Autodesk Inventor part; units mm, degrees
ref_plane "YZ Plane" through (0, 0, 0) normal (1, 0, 0) x (0, 1, 0)
ref_plane "XZ Plane" through (0, 0, 0) normal (0, 1, 0) x (-1, 0, 0)
ref_plane "XY Plane" through (0, 0, 0) normal (0, 0, 1) x (1, 0, 0)
sketch "Sketch1" plane through (0, 0, 0) normal (0, 1, 0) x (-1, 0, 0)
  line L0 (75, 59) -> (-75, 59)
  line L1 (-75, 59) -> (-75, -59)
  line L2 (-75, -59) -> (75, -59)
  line L3 (75, -59) -> (75, 59)
  line L4 (75, 59) -> (-75, -59) construction
  line L5 (-75, 59) -> (75, -59) construction
  line L6 (62.0096, 59) -> (62.0096, -65)
  line L7 (105, 0) -> (-105, 0)
  line L8 (0, -90) -> (0, 85)
  line L9 (-62.0096, 59) -> (-62.0096, -65)
  line L10 (61.6096, 59) -> (61.6096, -59)
  line L11 (-61.6096, 59) -> (-61.6096, -59)
  line L12 (-71, 55) -> (71, 55)
  line L13 (71, 55) -> (71, -55)
  line L14 (71, -55) -> (-71, -55)
  line L15 (-71, -55) -> (-71, 55)
  line L16 (61.6096, 55) -> (53.6096, 55)
  line L17 (53.6096, 55) -> (53.6096, 47)
  line L18 (53.6096, 47) -> (61.6096, 47)
  line L19 (61.6096, 47) -> (61.6096, 55)
  line L20 (61.6096, -55) -> (53.6096, -55)
  line L21 (53.6096, -55) -> (53.6096, -47)
  line L22 (53.6096, -47) -> (61.6096, -47)
  line L23 (-61.6096, 55) -> (-53.6096, 55)
  line L24 (-53.6096, 55) -> (-53.6096, 47)
  line L25 (-53.6096, 47) -> (-61.6096, 47)
  line L26 (-61.6096, 47) -> (-61.6096, 55)
  line L27 (-53.6096, -55) -> (-53.6096, -47)
  line L28 (-53.6096, -47) -> (-61.6096, -47)
  line L29 (-61.6096, -55) -> (-53.6096, -55)
  line L30 (-61.6096, 12) -> (-53.6096, 12)
  line L31 (-53.6096, 12) -> (-53.6096, 20)
  line L32 (-53.6096, 20) -> (-61.6096, 20)
  line L33 (-61.6096, 20) -> (-61.6096, 12)
  line L34 (-61.6096, -12) -> (-53.6096, -12)
  line L35 (-53.6096, -12) -> (-53.6096, -20)
  line L36 (-53.6096, -20) -> (-61.6096, -20)
  circle A0 centre (57.6096, 51) radius 1.55
  line L37 (61.6096, 51) -> (53.6096, 51)
  line L38 (57.6096, 55) -> (57.6096, 47)
  circle A1 centre (57.6096, -51) radius 1.55
  circle A2 centre (-57.6096, 51) radius 1.55
  circle A3 centre (-57.6096, -51) radius 1.55
  line L39 (-53.6096, 16) -> (-61.6096, 16)
  line L40 (-57.6096, 20) -> (-57.6096, 12)
  circle A4 centre (-57.6096, 16) radius 1.55
  circle A5 centre (-57.6096, -16) radius 1.55
  line L41 (53.6096, 51) -> (-53.6096, 51)
  line L42 (57.6096, 47) -> (57.6096, -47)
  line L43 (53.6096, -51) -> (-53.6096, -51)
  line L44 (-57.6096, -47) -> (-57.6096, -20)
  line L45 (-57.6096, -12) -> (-57.6096, 12)
  line L46 (-57.6096, 20) -> (-57.6096, 47)
  line L47 (53.6096, 47) -> (-53.6096, -47)
  line L48 (-53.6096, 47) -> (53.6096, -47)
  line L49 (0, 0) -> (57.6096, 0)
  line L50 (0, 0) -> (-57.6096, 0)
  line L51 (0, 0) -> (-53.6096, 16)
  line L52 (0, 0) -> (-53.6096, -16)
  circle A6 centre (0, 0) radius 6
  line L53 (53.6096, 48.9948) -> (3.3795, 4.9577)
  line L54 (53.6096, 52.5) -> (-53.6096, 52.5)
  line L55 (59.1096, 47) -> (59.1096, -47)
  line L56 (53.6096, -52.5) -> (-53.6096, -52.5)
  line L57 (-59.1096, -47) -> (-59.1096, -20)
  line L58 (-59.1096, -12) -> (-59.1096, 12)
  line L59 (-59.1096, 20) -> (-59.1096, 47)
  line L60 (-55.885, 47) -> (-5.3572, 2.7019)
  line L61 (-5.9958, 0.2241) -> (-53.6096, 14.4346)
  line L62 (-53.6096, -17.5654) -> (-5.1378, -3.0988)
  line L63 (-3.3795, -4.9577) -> (-53.6096, -48.9948)
  line L64 (5.8095, -1.5) -> (57.6096, -1.5)
  line L65 (56.1096, 47) -> (56.1096, -47)
  line L66 (53.6096, 49.5) -> (-53.6096, 49.5)
  line L67 (55.5873, 46.739) -> (5.3572, 2.7019)
  line L68 (5.8095, 1.5) -> (57.6096, 1.5)
  line L69 (-53.9073, 49.2558) -> (-3.3795, 4.9577)
  line L70 (-5.1378, 3.0988) -> (-52.7517, 17.3093)
  line L71 (-5.3572, -2.7019) -> (-55.5873, -46.739)
  line L72 (53.6096, -49.5) -> (-53.6096, -49.5)
  line L73 (-56.1096, -47) -> (-56.1096, -20)
  line L74 (-56.1096, -12) -> (-56.1096, 12)
  line L75 (-56.1096, 20) -> (-56.1096, 47)
  line L76 (-54.4676, -14.6907) -> (-5.9958, -0.2241)
  line L77 (3.3795, -4.9577) -> (53.6096, -48.9948)
  line L78 (5.3572, -2.7019) -> (55.5873, -46.739)
  line L79 (1.5, 49.5) -> (1.5, 5.8095)
  line L80 (-1.5, 49.5) -> (-1.5, 5.8095)
  line L81 (1.5, -49.5) -> (1.5, -5.8095)
  line L82 (-1.5, -49.5) -> (-1.5, -5.8095)
  line L83 (-52.7517, 17.3093) -> (-53.6096, 17.5654)
  line L84 (55.5873, -46.739) -> (55.885, -47)
  line L85 (55.5873, 46.739) -> (55.885, 47)
  line L86 (-55.5873, -46.739) -> (-58.8433, -49.5936)
  point P0 (-53.6096, 55)
  point P1 (-61.6096, 55)
  point P2 (-61.6096, 47)
  point P3 (-61.6096, 0)
  point P4 (-71, 0)
  point P5 (53.6096, 55)
  point P6 (4.5116, -3.9554)
  point P7 (56.1096, -1.5)
  point P8 (-4.5116, -3.9554)
  point P9 (-56.1096, -20)
  point P10 (1.5, -49.5)
  point P11 (1.5, -5.8095)
  point P12 (-1.5, -5.8095)
  point P13 (-1.5, -49.5)
  point P14 (-1.5, 5.8095)
  point P15 (-3.3795, 4.9577)
  point P16 (-53.6096, 48.9948)
  point P17 (-1.5, 49.5)
  point P18 (56.1096, 1.5)
  point P19 (4.5116, 3.9554)
  point P20 (-53.6096, -14.4346)
  point P21 (-5.7494, 1.7159)
  point P22 (-61.6096, -47)
  point P23 (-61.6096, -55)
  point P24 (-53.6096, -55)
  point P25 (53.6096, -55)
  point P26 (61.6096, -55)
  point P27 (61.6096, -47)
  point P28 (61.6096, 47)
  point P29 (5.3572, -2.7019)
  point P30 (-55.885, -47)
  point P31 (-6.1568, -3.4029)
  point P32 (5.3572, 2.7019)
  point P33 (-6.1568, 3.4029)
  dimension "d13" = 12
  dimension "d0" = 150
  dimension "d1" = 118
  dimension "d2" = 12.9904
  dimension "d3" = 0.4
  dimension "d4" = 4
  dimension "d5" = 8
  dimension "d6" = 8
  dimension "d7" = 8
  dimension "d8" = 8
  dimension "d9" = 12
  dimension "d10" = 3.1
  dimension "d11" = 3.1
  dimension "d14" = 3
  dimension "d15" = 3
  dimension "d16" = 3
  dimension "d17" = 3
  dimension "d18" = 3
  dimension "d19" = 3
  dimension "d20" = 3
  dimension "d21" = 3
  dimension "d22" = 3
  dimension "d23" = 3
  dimension "d24" = 3
  dimension "d25" = 3
extrude "Extrusion1" add sketch "Sketch1" along normal blind 3 contours L10 L37 A0 L38 L12 | L10 L18 L38 A0 L37 | L38 A0 L37 L17 L12 | L12 L24 L25 L11 | L54 L17 L41 L8 | L8 L41 L24 L54 | L14 L21 L22 L10 | L55 L22 L42 L7 | L7 L42 L18 L55 | L41 L17 L66 L8 | L8 L66 L24 L41 | L38 L18 L17 L37 A0 | L42 L64 L65 L7 | L7 L65 L68 L42 | L32 L40 A4 L39 L11 | L25 L46 L32 L59 | L66 L79 A6 L8 | L8 A6 L80 L66 | L42 L68 L65 L18 | L56 L8 L43 L21 | L65 L64 A6 L7 | L7 A6 L68 L65 | L42 L22 L65 L64 | L11 L28 L27 L14 | L56 L27 L43 L8 | L39 A4 L40 L30 L11 | L25 L75 L32 L46 | A6 L47 L8 | L8 L48 A6 | L43 L8 L72 L21 | A6 L48 L7 | L7 L47 A6 | L43 L27 L72 L8 | L58 L30 L45 L7 | L7 L45 L34 L58 | L34 L35 L36 L11 | L32 L31 L39 A4 L40 | L52 A6 L7 | L48 A6 L8 | L8 A6 L47 | L51 A6 L48 | L7 A6 L51 | L47 A6 L52 | L17 L47 A6 L53 | L69 A6 L48 L24 | L85 L67 A6 L47 L18 | L22 L48 A6 L78 L84 | L57 L36 L44 L28 | L72 L82 A6 L8 | L8 A6 L81 L72 | L45 L30 L74 L7 | L7 L74 L34 L45 | A4 L39 L31 L30 L40 | L25 L48 A6 L70 L60 | A6 L63 L27 L47 | L47 L28 L86 L71 L62 A6 | L48 L21 L77 A6 | A6 L61 L31 L51 | L51 L31 L83 L70 L60 A6 | A6 L71 L62 L35 L52 | L52 L35 L76 A6 | L44 L36 L73 L28 | L70 A6 L60 | L62 L71 A6
equation "\"d0\" = BodyLength"
equation "\"d1\" = BodyWidth"
equation "\"d2\" = 0.433013 * BodyHeight"
equation "\"d4\" = SideThickness"
equation "\"d5\" = M3ScrewInsertBrim"
equation "\"d6\" = M3ScrewInsertBrim"
equation "\"d7\" = M3ScrewInsertBrim"
equation "\"d8\" = M3ScrewInsertBrim"
equation "\"d10\" = M3ScrewDia"
equation "\"d11\" = M3ScrewDia"
equation "\"SideThickness_1\" = 4"
equation "\"M3ScrewInsertBrim_1\" = 8"
equation "\"M3ScrewDia_1\" = 3.1"
properties part number "HexScrewGuideV2"
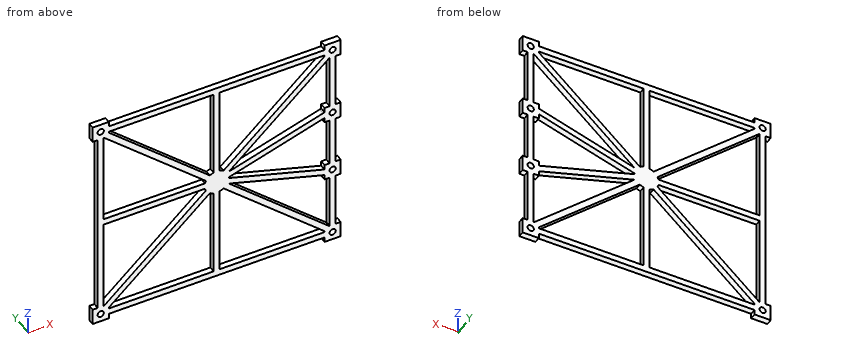
Part model, mm, in its own coordinate system. Coordinates: 2 decimals unless noted, no trailing zeros. Order: outer loops, then holes, each group sorted by start corner. A loop starts at its lowest first (then second) coordinate and runs counter-clockwise, first axis right, second up.
(1) Slice it at D-D, the plane x = 26. Write the cut outline in (y, z), and give its area (3 significant figures).
Check sheet entries:
outline: (0, -52.5) - (3, -52.5) - (3, -49.5) - (0, -49.5) - close; (0, -24.79) - (3, -24.79) - (3, -20.8) - (0, -20.8) - close; (0, -9.33) - (3, -9.33) - (3, -6.19) - (0, -6.19) - close; (0, 6.19) - (3, 6.19) - (3, 9.33) - (0, 9.33) - close; (0, 20.8) - (3, 20.8) - (3, 24.79) - (0, 24.79) - close; (0, 49.5) - (3, 49.5) - (3, 52.5) - (0, 52.5) - close
area: 60.7 mm2
(2) Slice it at C-C, the plane z = 22. Write the cut outline in (x, y), and give its area (3 significant figures).
Check sheet entries:
outline: (-59.11, 0) - (-56.11, 0) - (-56.11, 3) - (-59.11, 3) - close; (-27.37, 0) - (-22.82, 0) - (-22.82, 3) - (-27.37, 3) - close; (-1.5, 0) - (1.5, 0) - (1.5, 3) - (-1.5, 3) - close; (22.82, 0) - (27.37, 0) - (27.37, 3) - (22.82, 3) - close; (56.11, 0) - (59.11, 0) - (59.11, 3) - (56.11, 3) - close
area: 54.3 mm2
(3) Slice it at A-A, the plane z = -51. Write the cut outline in (x, y), and give its area (3 significant figures).
Check sheet entries:
outline: (-61.61, 0) - (-59.16, 0) - (-59.16, 3) - (-61.61, 3) - close; (-56.06, 0) - (56.06, 0) - (56.06, 3) - (-56.06, 3) - close; (59.16, 0) - (61.61, 0) - (61.61, 3) - (59.16, 3) - close
area: 351 mm2
(4) Pin check, flat tips, straight feed: pin 1 Ø0.9 at (y, z) = (2, 17) entering from -X; pin 2 Ø1.5 at (y, z) = (1, -37) entering from +X; pin 3 Ø1.5 at (x, y) = (16.5, 1) entering from -Z. Stop position of each tip, or through.
Check sheet entries:
pin 1: stops at x = -59.11
pin 2: stops at x = 59.11
pin 3: stops at z = -52.5
(5) Probe L1, parallel to Z at x = 46.5, y = 0.55; L2, parallel to X at y = 1.95, z = -37.5; L3, parallel to Z at x = 17.5, y = 0.5. List the from-to ranges inside material, lowest first.
Check sheet entries:
L1: z = -52.5 to -49.5, -42.76 to -38.77, -15.44 to -12.31, 12.31 to 15.44, 38.77 to 42.76, 49.5 to 52.5
L2: x = -59.11 to -56.11, -45.05 to -40.5, -1.5 to 1.5, 40.5 to 45.05, 56.11 to 59.11
L3: z = -52.5 to -49.5, -17.34 to -13.35, -6.79 to -3.66, 3.66 to 6.79, 13.35 to 17.34, 49.5 to 52.5
(6) Slice it at B-B, the plane x = -32. Write the cut outline in (y, z).
Check sheet entries:
outline: (0, -52.5) - (3, -52.5) - (3, -49.5) - (0, -49.5) - close; (0, -30.05) - (3, -30.05) - (3, -26.06) - (0, -26.06) - close; (0, -1.5) - (3, -1.5) - (3, 1.5) - (0, 1.5) - close; (0, 26.06) - (3, 26.06) - (3, 30.05) - (0, 30.05) - close; (0, 49.5) - (3, 49.5) - (3, 52.5) - (0, 52.5) - close
